from build123d import *

# Parameters (mm, degrees)
SKETCH1_R           = 20
SKETCH1_R_2         = 2.1
BOSS_EXTRUDE1_DEPTH = 5
FILLET1_R           = 50
FILLET2_R           = 60
FILLET3_R           = 15


with BuildPart() as part:
    # Sketch1 → Boss-Extrude1 (new body)
    with BuildSketch(Plane.XY):
        Polygon((-80, 26.564623636), (-80, 86.564623636), (0, 86.564623636), (21.006226146, 86.564623636), (65.812994389, -36.540960351), (9.431437142, -57.06216895), (-21.006226146, 26.564623636), align=None)
        with Locations((20.5212086, 0.183066389)):
            Circle(SKETCH1_R, mode=Mode.SUBTRACT)
        with Locations((-67.5, 81.564623636)):
            Circle(SKETCH1_R_2, mode=Mode.SUBTRACT)
        with Locations((-67.5, 56.564623636)):
            Circle(SKETCH1_R_2, mode=Mode.SUBTRACT)
        with Locations((-67.5, 31.564623636)):
            Circle(SKETCH1_R_2, mode=Mode.SUBTRACT)
        with Locations((-29.5, 81.564623636)):
            Circle(SKETCH1_R_2, mode=Mode.SUBTRACT)
        with Locations((-29.5, 56.564623636)):
            Circle(SKETCH1_R_2, mode=Mode.SUBTRACT)
        with Locations((-29.5, 31.564623636)):
            Circle(SKETCH1_R_2, mode=Mode.SUBTRACT)
    extrude(amount=BOSS_EXTRUDE1_DEPTH)

    # Fillet1
    fillet1_edges = [part.edges().sort_by_distance(p)[0] for p in [
        (21.006226146, 86.564623636, 2.5),
    ]]
    fillet(fillet1_edges, radius=FILLET1_R)

    # Fillet2
    fillet2_edges = [part.edges().sort_by_distance(p)[0] for p in [
        (-21.006226146, 26.564623636, 2.5),
    ]]
    fillet(fillet2_edges, radius=FILLET2_R)

    # Fillet3
    fillet3_edges = [part.edges().sort_by_distance(p)[0] for p in [
        (65.812994389, -36.540960351, 2.5),
        (9.431437142, -57.06216895, 2.5),
    ]]
    fillet(fillet3_edges, radius=FILLET3_R)


solid = part.part
Geometry check sheet. Reference: the model listing, model coordinates, mm. Give positions to 0.01 mm unless a question says otherwise; leave off trailing zeros. Loops run counter-clockwise (first coordinate to the right, second up) from the corner with the lowest first, then second, coordinate; pieces in that order, holes last. Notation, with made-up numbers: M -27.75,83 L -15.75,83 A7 cw -15.75,94 Z; hole C 26.5,82 d11. An arc over 180 degrees is marked long. Answer as a JSON object with one key per item and string values. Group by question number.
Item 1: Sectioned sample at B-B on y = 13.5. Record the boundary of the cut face in (x, z), plus the area to 3 significant figures.
Item 2: Material ranges on L1, parallel to Y at x = -67.5, z = 2.95; L2, parallel to X at y = 57.5, z = 4.5; L3, parallel to Y at x = -29.5, z = 1.2, recorded low to high.
Item 3: Mould release check, pull along Y, two halves, no side actions. Record for faces 1 (the cylindrical face through (60.111, -34.064, 2.535)), 2 (the flat face through (-71, 26.565, 2)), 3 (the cylindrical face through (-29.955, 79.515, 2.465)): pulls with the +Y half, pulls with the -Y half, needs draft (parallel to the pull), parting line crosses it, or undercut.
Item 4: Sectioned sample at D-D on x = 17. Record the boundary of the cut face in (y, z), plus the area to 3 significant figures.
Item 5: Gauge pin test, flat ends, axial feed: pin 1 (2 mm diameter, centred on y = 47, z = 3.5, fed in from +X); pin 2 (1.5 mm diameter, centred on x = 6.5, z = 1.5, fed in from -Y). Record the tip position at first contact, or that the pin passes through.
Item 6: Sectioned sample at C-C on z = 3.7. Record the boundary of the cut face in (x, y), plus the area to 3 significant figures.
Item 7: Sectioned sample at A-A on x = -67.5. Record the boundary of the cut face in (y, z), plus the area to 3 significant figures.
Findings below:
{
 "1": {"outline": "M -25.64,0 L 5.6,0 L 5.6,5 L -25.64,5 Z; M 35.44,0 L 47.6,0 L 47.6,5 L 35.44,5 Z", "area": "217 mm2"},
 "2": {"L1": "26.56 to 29.46, 33.66 to 54.46, 58.66 to 79.46, 83.66 to 86.56", "L2": "-80 to -69.38, -65.62 to -31.38, -27.62 to 31.4", "L3": "16.33 to 29.46, 33.66 to 54.46, 58.66 to 79.46, 83.66 to 86.56"},
 "3": {"face 1": "parting line crosses it", "face 2": "pulls with the -Y half", "face 3": "undercut"},
 "4": {"outline": "M -52.77,0 L -19.5,0 L -19.5,5 L -52.77,5 Z; M 19.87,0 L 75.79,0 L 75.79,5 L 19.87,5 Z", "area": "446 mm2"},
 "5": {"pin 1": "x = 35.77", "pin 2": "y = -47.87"},
 "6": {"outline": "M -80,26.56 L -63.02,26.56 A60 cw -6.64,-12.91 L 4.3,-42.97 A15 ccw 23.53,-51.93 L 51.72,-41.67 A15 ccw 60.68,-22.45 L 32.98,53.67 A50 ccw -14,86.56 L -80,86.56 Z; hole C -67.5,31.56 d4.2; hole C -67.5,56.56 d4.2; hole C -67.5,81.56 d4.2; hole C -29.5,31.56 d4.2; hole C -29.5,56.56 d4.2; hole C -29.5,81.56 d4.2; hole C 20.52,0.18 d40", "area": "10,100 mm2"},
 "7": {"outline": "M 26.56,0 L 29.46,0 L 29.46,5 L 26.56,5 Z; M 33.66,0 L 54.46,0 L 54.46,5 L 33.66,5 Z; M 58.66,0 L 79.46,0 L 79.46,5 L 58.66,5 Z; M 83.66,0 L 86.56,0 L 86.56,5 L 83.66,5 Z", "area": "237 mm2"}
}
